Read the model definition and answer for the solid it produces. Units are mm, in the model's axes. Face numbers are marked on the shaded views. Coordinates: 2 decimals unless noted, no trailing zeros. Order: outer loops, then holes, each group sorted by start corner. A loop starts at its lowest first (then second) coordinate and runs counter-clockwise, first axis right, second up. Notation, with made-up numbers: (-8.75, 0.5) - (39.25, 0.5) arc R21 ccw to (39.25, 14.5) - close; hole circle Ø1 at (-10, 16). An arc over 180 degrees is marked (long way). Use one line per item in the form item = value. Start each with the question number.
Autodesk Inventor part; units mm, degrees
ref_plane "YZ Plane" through (0, 0, 0) normal (1, 0, 0) x (0, 1, 0)
ref_plane "XZ Plane" through (0, 0, 0) normal (0, 1, 0) x (-1, 0, 0)
ref_plane "XY Plane" through (0, 0, 0) normal (0, 0, 1) x (1, 0, 0)
sketch "Sketch1" plane through (0, 0, 0) normal (0, 0, 1) x (1, 0, 0)
  line L0 (-19.225, 0) -> (-22.225, 0)
  line L1 (-22.225, 0) -> (-22.225, 380)
  line L2 (-22.225, 380) -> (-19.225, 380)
  line L3 (-19.225, 380) -> (-19.225, 0)
  line L4 (0, -86) -> (0, 481)
  line L5 (-19.225, 380) -> (-20.225, 380)
  line L6 (-20.225, 380) -> (-20.225, 400)
  line L7 (-20.225, 400) -> (-19.225, 400)
  line L8 (-19.225, 400) -> (-19.225, 380)
  line L9 (-19.225, 0) -> (-20.225, 0)
  line L10 (-20.225, 0) -> (-20.225, -5)
  line L11 (-20.225, -5) -> (-19.225, -5)
  line L12 (-19.225, -5) -> (-19.225, 0)
  point P0 (0, 0)
  point P1 (-20.225, 0)
  dimension "d0" = 22.225
  dimension "d1" = 3
  dimension "d2" = 380
  dimension "d4" = 1
  dimension "d5" = 20
  dimension "d6" = 1
  dimension "d7" = 5
revolve "Revolution1" add sketch "Sketch1" angle 360 about axis through (0, -10, 0) along (0, 1, 0)
properties part number "BodyCylinder" material "Brass"
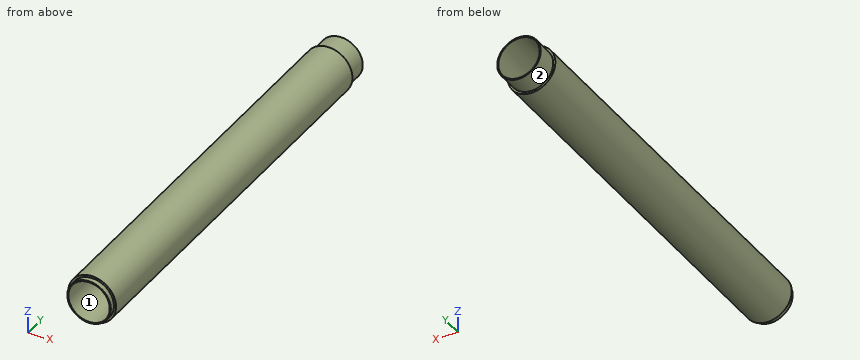
Q1. Given P1, Ø6, axis at y = 111.5, z = -16, coming from the +X side; P2, Ø10, axis at y = 294.5, z = -16, coming from the -X side; P3, Ø10, axis at x = -7.5, y = 341.5, coming from the -Z side, each flat-ended and moving along its own axis, determine where each tip first touches the part or whether it passes through.
Q2. Consider probe 1 along Z at (x, y) = (0, 193) (3 decimals); probe 2 along X at (y, z) = (290.5, 10.5); probe 3 along X at (y, z) = (281.5, 4). Determine where each line is inside the solid, lowest interval first.
Q3. A cutting plane is placed at C-C (y = 35). Give the vertices of the cut face in (x, z) (3 decimals), then the cut area to 3 significant figures.
Q4. For a pull along Z with two mould halves and no side action, classify the marked faces 1 and 2 as +Z half, -Z half, draft (parallel to the pull), parting line (faces both ways), or undercut.
Q5. A cutting plane is placed at B-B (z = 0). Give the vertices of the cut face in (x, y) (3 decimals), then the cut area to 3 significant figures.
Q6. A cutting plane is placed at A-A (x = 0). Give the vertices of the cut face in (y, z) (3 decimals), then the cut area to 3 significant figures.
Result sheet:
q1.P1 = 18.03
q1.P2 = -19.31
q1.P3 = -22.08
q2.probe_1 = -22.225 to -19.225, 19.225 to 22.225
q2.probe_2 = -19.59 to -16.1, 16.1 to 19.59
q2.probe_3 = -21.86 to -18.8, 18.8 to 21.86
q3.outline = circle Ø44.45 at (0, 0); hole circle Ø38.45 at (0, 0)
q3.area = 391 mm^2
q4.face_1 = undercut
q4.face_2 = parting line
q5.outline = (-22.225, 0) - (-20.225, 0) - (-20.225, -5) - (-19.225, -5) - (-19.225, 400) - (-20.225, 400) - (-20.225, 380) - (-22.225, 380) - close; (19.225, -5) - (20.225, -5) - (20.225, 0) - (22.225, 0) - (22.225, 380) - (20.225, 380) - (20.225, 400) - (19.225, 400) - close
q5.area = 2,330 mm^2
q6.outline = (-5, -20.225) - (0, -20.225) - (0, -22.225) - (380, -22.225) - (380, -20.225) - (400, -20.225) - (400, -19.225) - (-5, -19.225) - close; (-5, 19.225) - (400, 19.225) - (400, 20.225) - (380, 20.225) - (380, 22.225) - (0, 22.225) - (0, 20.225) - (-5, 20.225) - close
q6.area = 2,330 mm^2
